The drawing under review shows one solid part. Ordinate dimensions are in mm from its lowest x, y, z. A direction names the side the tool comes from. Round coordinates to 2 decimals unless told otherwise and drop trailing zeros. Order: outer loops, then holes, each group sorted by start corner. A loop starts at its lowest first (then second) coordinate and runs counter-clockwise, first axis right, second up. Notation, with made-up numbers: M 35.25,41 L 57.25,41 A16 ccw 57.25,55 Z; hole C 62.5,69 d11. An arc over 180 degrees is marked long. Use a Markdown table: item, result.
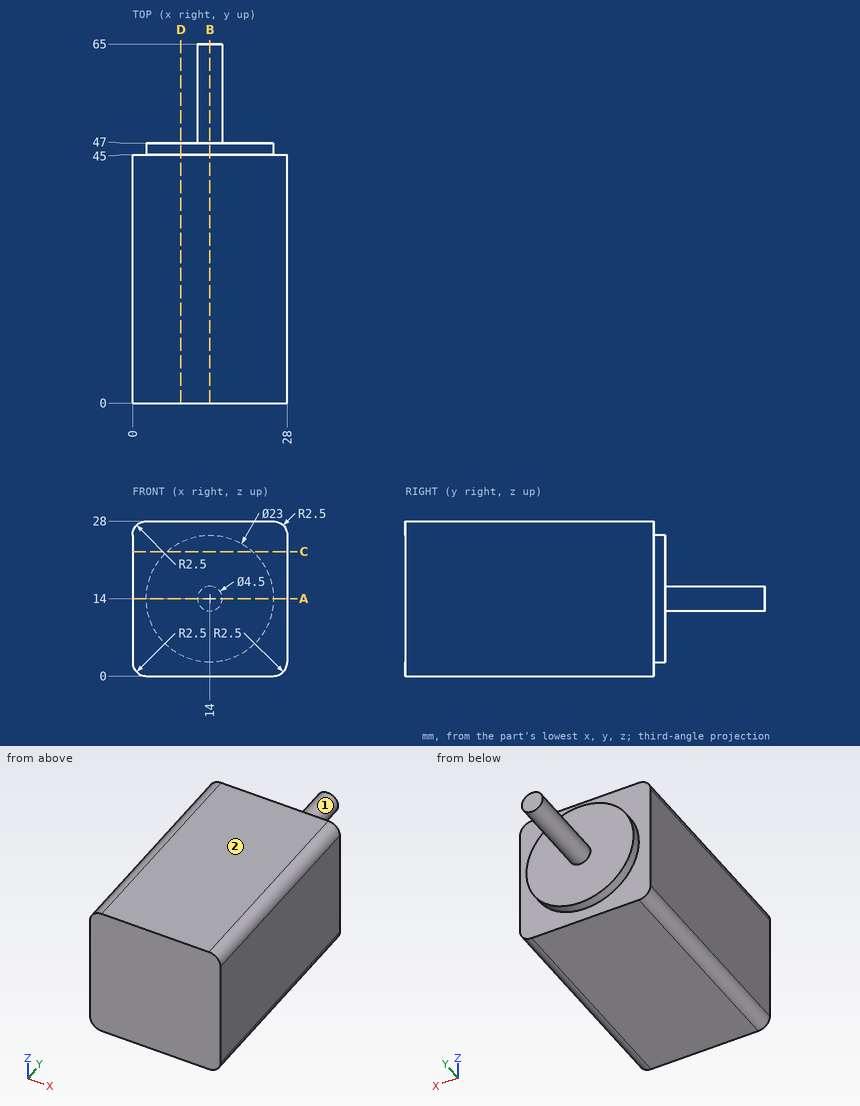
Q1. Add section C-C (z = 22.5). Write out the cut boundary in (x, y), then the cut area to 3 significant figures.
Determined:
| item | result |
|---|---|
| outline | M 0,0 L 28,0 L 28,45 L 21.75,45 L 21.75,47 L 6.25,47 L 6.25,45 L 0,45 Z |
| area | 1,290 mm^2 |
Q2. Wall thickness on line 1 along Y through (x, z) = (9, 15); line 2 along Y through (x, z) = (3, 9.5); line 3 along X through (y, z) = (24.5, 2.25): over which ranges is each line inside the solid? List them lowest first. Write a range as [from, to].
Determined:
| item | result |
|---|---|
| line 1 | y = [0, 47] |
| line 2 | y = [0, 45] |
| line 3 | x = [0.01, 27.99] |
Q3. Clearance check with flat-ended pins moving along their axes: pin 1 (8 mm diameter, centred on y = 56, z = 22, fed in from -X); pin 2 (12 mm diameter, centred on y = 56, z = 6, fed in from +X); pin 3 (2 mm diameter, centred on x = 3, z = 13, fed in from +Y). State where each tip first meets the part, or that it passes through.
Determined:
| item | result |
|---|---|
| pin 1 | passes through |
| pin 2 | stops at x = 15.03 |
| pin 3 | stops at y = 47 |
Q4. Machinability: for the marked faces 1 and 2, which of the approach directions +Z, -Z, +X, -X, +Y, -Y give a long, thin tool a straight path to every point of the face, cutting with its end or side? Answer none if there is none.
Determined:
| item | result |
|---|---|
| face 1 | +Y |
| face 2 | +Z, +X, -X, +Y, -Y |
Q5. Add section A-A (z = 14). Write out the cut boundary in (x, y), then the cut area to 3 significant figures.
Determined:
| item | result |
|---|---|
| outline | M 0,0 L 28,0 L 28,45 L 25.5,45 L 25.5,47 L 16.25,47 L 16.25,65 L 11.75,65 L 11.75,47 L 2.5,47 L 2.5,45 L 0,45 Z |
| area | 1,390 mm^2 |
Q6. Add section B-B (x = 14). Write out the cut boundary in (y, z).
Determined:
| item | result |
|---|---|
| outline | M 0,0 L 45,0 L 45,2.5 L 47,2.5 L 47,11.75 L 65,11.75 L 65,16.25 L 47,16.25 L 47,25.5 L 45,25.5 L 45,28 L 0,28 Z |
Q7. Add section D-D (x = 8.75). Write out the cut boundary in (y, z).
Determined:
| item | result |
|---|---|
| outline | M 0,0 L 45,0 L 45,3.77 L 47,3.77 L 47,24.23 L 45,24.23 L 45,28 L 0,28 Z |
